Verification items for the finished model (mm, model axes). Face numbers are marked on the shaded views. A direction names the side the tool comes from. Coordinates: 2 decimals unless noted, no trailing zeros. Write each loop counter-clockwise with the first axis right and the second up, starting at its lowest first coordinate (ties: lowest second). Pieces come first, ordered by that corner, then holes. Notation, with made-up numbers: M -0.5,34 L 51.5,34 A24 ccw 51.5,68 Z; hole C -36,13 d10. An arc over 180 degrees is marked long. One line per item, written item: value.
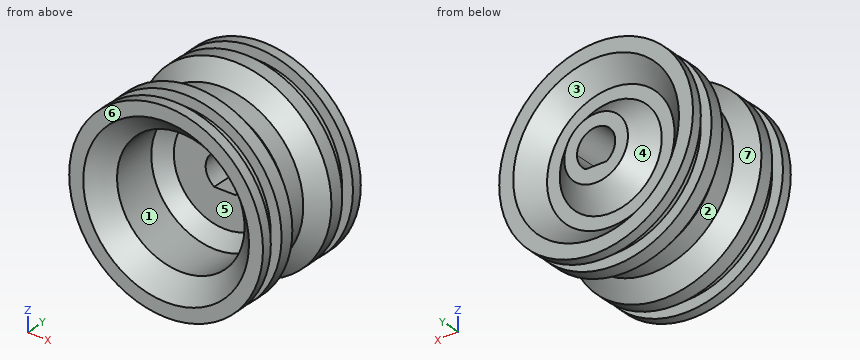
```python
from build123d import *

# Parameters (mm, degrees)
SKETCH_1_R          = 15.2
EXTRUDE_1_DEPTH     = 10
SKETCH_2_W          = 1.7
SKETCH_2_H          = 2.2
SKETCH_4_R          = 10
CUT_EXTRUDE_1_DEPTH = 12
CUT_EXTRUDE_2_DEPTH = 15
CHAMFER_1_SIZE      = 3
CUT_EXTRUDE_START   = -3
SKETCH_6_R          = 10
SKETCH_6_R_2        = 5
CUT_EXTRUDE_3_DEPTH = 3
CHAMFER_2_SIZE      = 3
SKETCH_7_W          = 2.5
SKETCH_7_H          = 8
CHAMFER_3_SIZE      = 2.5
CHAMFER_4_SIZE      = 2


with BuildPart() as part:
    # 草图1 → 凸台-拉伸1 (new, symmetric)
    with BuildSketch(Plane(origin=(0, 0, 0), x_dir=(1, 0, 0), z_dir=(0, 1, 0))):
        with Locations(Location((0, 0, 0), (0, 0, 270))):
            Circle(SKETCH_1_R)
    extrude(amount=EXTRUDE_1_DEPTH, both=True)

    # 草图2 → 切除-旋转1 (revolve, cut)
    with BuildSketch(Plane.XY, mode=Mode.PRIVATE) as cut_revolve_1_sk:
        with Locations((14.35, 7.3)):
            Rectangle(SKETCH_2_W, SKETCH_2_H)
    cut_revolve_1 = revolve(cut_revolve_1_sk.sketch.rotate(Axis((0, 8.4, 0), (0, -1, 0)), 90), axis=Axis((0, 8.4, 0), (0, -1, 0)), mode=Mode.SUBTRACT)

    # 镜向1: 切除-旋转1 across plane
    add(cut_revolve_1.mirror(Plane.ZX), mode=Mode.SUBTRACT)

    # 草图4 → 切除-拉伸1 (cut)
    with BuildSketch(Plane.XZ.offset(10)):
        with Locations(Location((0, 0, 0), (0, 0, 270))):
            Circle(SKETCH_4_R)
    extrude(amount=-CUT_EXTRUDE_1_DEPTH, mode=Mode.SUBTRACT)

    # 草图5 → 切除-拉伸2 (cut)
    with BuildSketch(Plane(origin=(0, 10, 0), x_dir=(1, 0, 0), z_dir=(0, 1, 0))):
        with BuildLine():
            Line((1.658312395, 2.5), (-1.658312395, 2.5))
            ThreePointArc((-1.658312395, 2.5), (-1.418637165, -2.643382037), (3, 0))
            ThreePointArc((3, 0), (2.643382037, 1.418637165), (1.658312395, 2.5))
        make_face()
    extrude(amount=-CUT_EXTRUDE_2_DEPTH, mode=Mode.SUBTRACT)

    # 倒角1
    chamfer_1_edges = [part.edges().sort_by_distance(p)[0] for p in [
        (0, -10, 10),
    ]]
    chamfer(chamfer_1_edges, length=CHAMFER_1_SIZE)

    # 草图6 → 切除-拉伸3 (cut)
    with BuildSketch(Plane(origin=(0, 10, 0), x_dir=(1, 0, 0), z_dir=(0, 1, 0)).offset(CUT_EXTRUDE_START)):
        with Locations(Location((0, 0, 0), (0, 0, 90))):
            Circle(SKETCH_6_R)
        with Locations(Location((0, 0, 0), (0, 0, 270))):
            Circle(SKETCH_6_R_2, mode=Mode.SUBTRACT)
    extrude(amount=CUT_EXTRUDE_3_DEPTH, mode=Mode.SUBTRACT)

    # 倒角2
    chamfer_2_edges = [part.edges().sort_by_distance(p)[0] for p in [
        (0, 7, -5),
        (0, 10, 10),
    ]]
    chamfer(chamfer_2_edges, length=CHAMFER_2_SIZE - 0.0001)  # a hair under: the kernel refuses the full size

    # 草图7 → 切除-旋转2 (revolve, cut)
    with BuildSketch(Plane(origin=(0, 0, 0), x_dir=(0, 0, -1), z_dir=(1, 0, 0))):
        with Locations((13.95, 0)):
            Rectangle(SKETCH_7_W, SKETCH_7_H)
    revolve(axis=Axis((0, 2, 0), (0, 1, 0)), mode=Mode.SUBTRACT)

    # 倒角3
    chamfer_3_edges = [part.edges().sort_by_distance(p)[0] for p in [
        (0, -4, 12.7),
        (0, 4, 12.7),
    ]]
    chamfer(chamfer_3_edges, length=CHAMFER_3_SIZE - 0.0001)  # a hair under: the kernel refuses the full size

    # 倒角4
    chamfer_4_edges = [part.edges().sort_by_distance(p)[0] for p in [
        (0, 2, 10),
    ]]
    chamfer(chamfer_4_edges, length=CHAMFER_4_SIZE)


solid = part.part
```
Item 1: Cross-section at B-B, the plane y = 5.5. Enter the section's corners in (x, z), and give its area (3 significant figures).
The answers:
outline: C 0,0 d30.4; hole M -1.66,-2.5 L 1.66,-2.5 A3 ccw long Z
area: 699 mm²
Item 2: Scan lines: line 1 (Y direction, x = -2, z = 13.5); line 2 (X direction, y = -2.5, z = 0); line 3 (X direction, y = -6.25, z = 4). Record each from-to range of solid material in increasing order.
The answers:
line 1: y = -10 to -8.4, -6.2 to -2.45, 2.45 to 6.2, 8.4 to 10
line 2: x = -13.7 to -10, 10 to 13.7
line 3: x = -12.89 to -9.17, 9.17 to 12.89
Item 3: Access from +Z, -Z, +X, -X, +Y, -Y to the whole of each face (thin tool, end or side, straight path). Record for the marked faces 1, 2 and 3.
The answers:
face 1: -Y
face 2: none
face 3: +Y
Item 4: Draft check along Z on the marked faces 4, 5, 6 and 7. Enter one of: released by +Z, released by -Z, zero draft, split by the parting line, or undercut.
The answers:
face 4: undercut
face 5: undercut
face 6: zero draft
face 7: split by the parting line
Item 5: Cross-section at D-D, the plane y = 2.75. Enter the section's corners in (x, z).
The answers:
outline: C 0,0 d27.9; hole M -1.66,-2.5 L 1.66,-2.5 A3 ccw long Z
Item 6: Cross-section at C-C, the plane y = -8. Enter the section's corners in (x, z).
The answers:
outline: C 0,0 d27; hole C 0,0 d22
Item 7: Cross-section at A-A, the plane y = -0.75. Enter the section's corners in (x, z).
The answers:
outline: C 0,0 d25.4; hole C 0,0 d20
Item 8: Go/stop test with flat-tipped pins: P1, Ø10, axis at x = -8, y = -7, coming from the -Z side; P2, Ø8, axis at x = 6.5, y = 1, coming from the +Z side; P3, Ø6, axis at y = -7.5, z = -3.5, coming from the -X side. Record where each tip stops, or that it passes through.
The answers:
P1: stops at z = -14.89
P2: stops at z = 14.7
P3: stops at x = -15.19
